Part model, mm, in its own coordinate system. Face numbers are marked on the shaded views. A direction names the side the tool comes from. Coordinates: 2 decimals unless noted, no trailing zeros. Loops run counter-clockwise (first coordinate to the right, second up) from the corner with the lowest first, then second, coordinate; pieces in that order, holes last. Notation, with made-up numbers: (72, 54) -> (80, 54) arc R25 ccw to (80, 92) -> close; hole circle Ø3 at (77.5, 68.25). An arc over 180 degrees is marked (long way). One line per question, with ' | ' between items. Start each with the question number.
1) Cut at A-A (x = 88.9). List the corners of the cut face in (y, z).
2) Cut at C-C (z = 48). List the corners of the cut face in (x, y).
3) Probe L1, parallel to X at y = 44, z = 50; L2, parallel to X at y = 16.5, z = 36; L3, parallel to Y at x = -65.5, z = 22.5. List the from-to ranges inside material, lowest first. Write a range as from..to.
4) 3-axis set-ups, long thin cutter, end or side, ignore diameter. For the marked faces 1 and 2: which of +Z, -Z, +X, -X, +Y, -Y reach the whole face in a straight line?
5) Two-plate mould, pull along Y, no slides. Class the marked faces 3, 4 and 5: released by +Y, released by -Y, zero draft, split by the parting line, or undercut.
6) Drop flat-ended pins along their axis: pin 1 (20.5 mm diameter, centred on x = -36.5, z = 31.5, fed in from +Y); pin 2 (4 mm diameter, centred on x = 22, y = 58, fed in from -Z); pin 3 (1 mm diameter, centred on x = 4.5, z = 17, fed in from -Y). Give the stop position or say it passes through.
7) Cut at B-B (y = 11). List the corners of the cut face in (x, z).
8) Cut at D-D (x = -38.1). List the corners of the cut face in (y, z).
from build123d import *

# Parameters (mm, degrees)
SKETCH1_W                      = 254
SKETCH1_H                      = 127
RECTANGLE_PRISON_DEPTH         = 127
TOP_SQUARE_CUT_DEPTH           = 291.99355663
TOP_SQUARE_CUT_DEPTH_BACK      = 291.99355663
BUTTOM_TRI_CUT_DEPTH           = 291.99355663
BUTTOM_TRI_CUT_DEPTH_BACK      = 291.99355663
SKETCH8_R                      = 25.4
OUTER_CIRCLE_CUT_DEPTH         = 25.4
SKETCH9_R                      = 19.05
INNER_CIRCLE_CUT_DEPTH         = 168.52450567
SKETCH11_R                     = 12.7
TWO_CIRCLES_OUT_DEPTH          = 12.7
SKETCH12_R                     = 19.05
CIRCLE_CUT_IN_THE_MIDDLE_DEPTH = 191.5


with BuildPart() as part:
    # Sketch1 → Rectangle prison (new body)
    with BuildSketch(Plane(origin=(0, 0, 0), x_dir=(1, 0, 0), z_dir=(0, 1, 0))):
        Rectangle(SKETCH1_W, SKETCH1_H)
    extrude(amount=RECTANGLE_PRISON_DEPTH)

    # Sketch6 → Top square cut (cut, two sides: drawn at the far end of the back side and taken through both)
    with BuildSketch(Plane(origin=(127, 0, 0), x_dir=(0, 0, -1), z_dir=(1, 0, 0)).offset(-TOP_SQUARE_CUT_DEPTH_BACK)):
        Polygon((-357.480633142, 63.5), (-63.5, 63.5), (0, 63.5), (0, 127), (0, 420.980633142), (-415.751398465, 836.732031608), (-773.232031608, 479.251398465), align=None)
    extrude(amount=TOP_SQUARE_CUT_DEPTH + TOP_SQUARE_CUT_DEPTH_BACK, mode=Mode.SUBTRACT)

    # Sketch7 → Buttom tri cut (cut, two sides: drawn at the far end of the back side and taken through both)
    with BuildSketch(Plane(origin=(127, 0, 0), x_dir=(0, 0, -1), z_dir=(1, 0, 0)).offset(-BUTTOM_TRI_CUT_DEPTH_BACK)):
        Polygon((-207.875699233, -207.875699233), (0, 0), (63.5, 63.5), (271.375699233, 271.375699233), (687.127097698, -144.375699233), (207.875699233, -623.627097698), align=None)
    extrude(amount=BUTTOM_TRI_CUT_DEPTH + BUTTOM_TRI_CUT_DEPTH_BACK, mode=Mode.SUBTRACT)

    # Sketch8 → outer circle cut (cut)
    with BuildSketch(Plane(origin=(0, 63.5, 0), x_dir=(1, 0, 0), z_dir=(0, 1, 0))):
        with Locations(Location((-88.9, -32.658118373, 0), (0, 0, 270))):
            Circle(SKETCH8_R)
        with Locations(Location((88.9, -32.658118373, 0), (0, 0, 270))):
            Circle(SKETCH8_R)
    extrude(amount=-OUTER_CIRCLE_CUT_DEPTH, mode=Mode.SUBTRACT)

    # Sketch9 → inner circle cut (cut, through all)
    with BuildSketch(Plane(origin=(0, 38.1, 0), x_dir=(1, 0, 0), z_dir=(0, 1, 0))):
        with Locations(Location((-88.9, -32.658118373, 0), (0, 0, 270))):
            Circle(SKETCH9_R)
        with Locations(Location((88.9, -32.658118373, 0), (0, 0, 270))):
            Circle(SKETCH9_R)
    extrude(amount=-INNER_CIRCLE_CUT_DEPTH, mode=Mode.SUBTRACT)

    # Sketch11 → Two circles out (add)
    with BuildSketch(Plane(origin=(0, 63.5, 0), x_dir=(1, 0, 0), z_dir=(0, 1, 0))):
        with Locations(Location((-38.1, -30.71024924, 0), (0, 0, 270))):
            Circle(SKETCH11_R)
        with Locations(Location((38.1, -30.71024924, 0), (0, 0, 270))):
            Circle(SKETCH11_R)
    extrude(amount=TWO_CIRCLES_OUT_DEPTH)

    # Sketch12 → Circle cut in the middle (cut, through all)
    with BuildSketch(Plane(origin=(0, 0, 0), x_dir=(1, 0, 0), z_dir=(0, -0.7071067811865475, -0.7071067811865476))):
        with Locations(Location((0, -44.901280605, 0), (0, 0, 270))):
            Circle(SKETCH12_R)
    extrude(amount=-CIRCLE_CUT_IN_THE_MIDDLE_DEPTH, mode=Mode.SUBTRACT)


solid = part.part
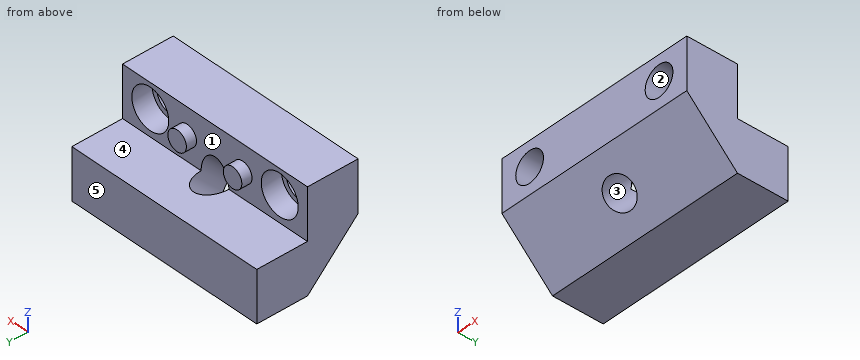
Reported:
1) outline: (0, 0) -> (63.5, -63.5) -> (127, -63.5) -> (127, 0) -> (63.5, 0) -> (63.5, 7.26) -> (38.1, 7.26) -> (38.1, 13.61) -> (0, 13.61) -> close; (0, 51.71) -> (38.1, 51.71) -> (38.1, 58.06) -> (63.5, 58.06) -> (63.5, 63.5) -> (0, 63.5) -> close
2) outline: (-127, 0) -> (-100.19, 0) -> (-100.19, 38.1) -> (-109.14, 38.1) -> (-109.14, 63.5) -> (-127, 63.5) -> close; (-77.61, 0) -> (77.61, 0) -> (77.61, 38.1) -> (68.66, 38.1) -> (68.66, 63.5) -> (-68.66, 63.5) -> (-68.66, 38.1) -> (-77.61, 38.1) -> close; (100.19, 0) -> (127, 0) -> (127, 63.5) -> (109.14, 63.5) -> (109.14, 38.1) -> (100.19, 38.1) -> close
3) L1: x = -127..-107.46, -70.34..70.34, 107.46..127 | L2: x = -127..-107.65, -70.15..70.15, 107.65..127 | L3: y = 0..63.5
4) face 1: +Y | face 2: +Y, -Y
5) face 3: undercut | face 4: zero draft | face 5: released by +Y
6) pin 1: stops at y = 76.2 | pin 2: stops at z = -60 | pin 3: stops at y = 0
7) outline: (-127, -11) -> (127, -11) -> (127, 63.5) -> (-127, 63.5) -> close; hole circle Ø38.1 at (-88.9, 32.66); hole circle Ø38.1 at (88.9, 32.66)
8) outline: (0, 0) -> (63.5, -63.5) -> (127, -63.5) -> (127, 0) -> (63.5, 0) -> (63.5, 18.01) -> (76.2, 18.01) -> (76.2, 43.41) -> (63.5, 43.41) -> (63.5, 63.5) -> (0, 63.5) -> close
